from build123d import *

# Parameters (mm, degrees)
F0_R     = 26.884522514
F1_DEPTH = 75
F2_T     = -2.5
F4_R     = 5


# Not quite as in the source:
# - a fillet or chamfer that OpenCascade refuses, or shapes differently, is made with other operations: its cross-section is extruded or revolved along the edge and cut away or added


with BuildPart() as f1:
    # F0 (on Top) → F1 (new body)
    with BuildSketch(Plane.XY):
        Circle(F0_R)
    extrude(amount=F1_DEPTH)

    # F2
    f2_openings = [f1.faces().sort_by_distance(p)[0] for p in [
        (0, 0, 75),
    ]]
    offset(amount=F2_T, openings=f2_openings)

    # F3: fillet of radius 5 on 1 edges, made by hand

    # F3_s1 → F3_t2 (revolve, cut)
    with BuildSketch(Plane.XZ):
        with BuildLine():
            ThreePointArc((26.884522514, 70.6698729811), (26.2146495329, 73.1698729811), (24.384522514, 75))
            Line((24.384522514, 75), (26.884522514, 75))
            Line((26.884522514, 75), (26.884522514, 70.6698729811))
        make_face()
    revolve(axis=Axis((0, 0, 75), (0, 0, 1)), mode=Mode.SUBTRACT)

    # F4
    f4_edges = [f1.edges().sort_by_distance(p)[0] for p in [
        (-26.884523, 0, 0),
    ]]
    fillet(f4_edges, radius=F4_R)


solid = f1.part
Check sheet for the modelled part. Datum: model origin and axes. Units: mm. Coordinates: 2 decimals unless noted, no trailing zeros. Loops run counter-clockwise (first coordinate to the right, second up) from the corner with the lowest first, then second, coordinate; pieces in that order, holes last. Notation, with made-up numbers: (0.25, -36.75) -> (26.25, -36.75) arc R9 ccw to (26.25, -22.75) -> close; hole circle Ø6 at (-1.75, -4.75). An arc over 180 degrees is marked (long way). Answer in a Markdown table with one row per item.
1. Material ranges on line 1 along Y through (x, z) = (0, 47); line 2 along Z through (x, y) = (14.5, 17); line 3 along Y through (x, z) = (19, 60), recorded low to high. Write a range as [from, to].
Check values:
| item | result |
|---|---|
| line 1 | y = [-26.88, -24.38], [24.38, 26.88] |
| line 2 | z = [0.02, 2.5] |
| line 3 | y = [-19.02, -15.28], [15.28, 19.02] |
2. Sectioned sample at C-C, the plane z = 60.5. Record the boundary of the cut face in (x, y), then the cut area to 3 significant figures.
Check values:
| item | result |
|---|---|
| outline | circle Ø53.77 at (0, 0); hole circle Ø48.77 at (0, 0) |
| area | 403 mm2 |
3. Sectioned sample at A-A, the plane x = 0. Record the boundary of the cut face in (y, z).
Check values:
| item | result |
|---|---|
| outline | (-26.88, 5) arc R5 ccw to (-21.88, 0) -> (21.88, 0) arc R5 ccw to (26.88, 5) -> (26.88, 70.67) arc R5 ccw to (24.38, 75) -> (24.38, 2.5) -> (-24.38, 2.5) -> (-24.38, 75) arc R5 ccw to (-26.88, 70.67) -> close |
4. Release check for a two-part mould opening along X. For faces 1 (the face through (0, 0, 2.5)), 2 (the face through (-17.97, 16.48, 38.24)), 3 (the face through (-5.828, -26.245, 37.375)), 4 (the face through (0, 0, 0)) record: released by +X, released by -X, zero draft, split by the parting line, or undercut.
Check values:
| item | result |
|---|---|
| face 1 | undercut |
| face 2 | undercut |
| face 3 | split by the parting line |
| face 4 | zero draft |
5. Go/stop test with flat-tipped pins: pin 1 (8 mm diameter, centred on x = -20.5, z = 38, fed in from +Y); pin 2 (10 mm diameter, centred on x = -13, z = 15.5, fed in from +Y); pin 3 (3 mm diameter, centred on y = -14, z = 36.5, fed in from -X). Record where each tip stops, or that it passes through.
Check values:
| item | result |
|---|---|
| pin 1 | stops at y = 21.23 |
| pin 2 | stops at y = 25.67 |
| pin 3 | stops at x = -23.8 |
